Check sheet for the modelled part. Datum: model origin and axes. Units: mm. Face numbers are marked on the shaded views. A direction names the side the tool comes from. Round coordinates to 2 decimals unless told otherwise and drop trailing zeros. Write each loop counter-clockwise with the first axis right and the second up, starting at its lowest first coordinate (ties: lowest second). Pieces come first, ordered by that corner, then holes. Notation, with made-up numbers: (11.5, 14.25) - (18.5, 14.25) arc R4 ccw to (18.5, 19.25) - close; hole circle Ø3 at (32, 76). An arc over 180 degrees is marked (long way). Answer as a JSON object with one key per item and string values. Group by question number.
Item 1: Sectioned sample at D-D on y = 7.25. Record the boundary of the cut face in (x, z), plus the area to 3 significant figures.
Item 2: Set-up check for the marked faces 1, 2 and 3: record each of +Z, -Z, +X, -X, +Y, -Y from which the full face is reachable in a straight line by a thin tool's end or side.
Item 3: Thickness scan on line 1 (X direction, y = 14, z = -38); line 2 (X direction, y = 11.5, z = -36); line 3 (Z direction, x = 34, y = 10.5). Record the ranges inside material, lowest first.
Item 4: Sectioned sample at A-A on y = 1. Record the boundary of the cut face in (x, z) (1 decimal), plus the area to 3 significant figures.
Item 5: Sectioned sample at B-B on z = -20. Record the boundary of the cut face in (x, y) (1 decimal), plus the area to 3 significant figures.
Item 6: Sectioned sample at C-C on x = 13.5. Record the boundary of the cut face in (y, z) (3 decimals), plus the area to 4 significant figures.
Item 7: Gauge pin test, flat ends, axial feed: P1, Ø5, axis at x = 51, y = 11, coming from the -Z side; P2, Ø6.5, axis at y = 7.5, z = -39, coming from the +X side; P3, Ø6.5, axis at x = 49.5, y = 11, coming from the +Z side. Record the tip position at first contact, or that the pin passes through.
```python
from build123d import *

# Parameters (mm, degrees)
SKETCH1_W               = 79.375
SKETCH1_H               = 79.375
BOSS_EXTRUDE1_DEPTH     = 4
SKETCH2_W               = 43.02
SKETCH2_H               = 43.02
SKETCH2_R               = 5.461
BOSS_EXTRUDE2_DEPTH     = 11
SKETCH3_R               = 5.461
CUT_EXTRUDE1_DEPTH      = 1
CUT_EXTRUDE1_DEPTH_BACK = 16
SKETCH4_W               = 38.805624494
SKETCH4_H               = 17.902161279
SKETCH4_W_2             = 9.122
SKETCH4_H_2             = 9.122
BOSS_EXTRUDE3_DEPTH     = 15


with BuildPart() as part:
    # Sketch1 → Boss-Extrude1 (new body)
    with BuildSketch(Plane(origin=(0, 0, 0), x_dir=(1, 0, 0), z_dir=(0, 1, 0))):
        with Locations((39.6875, 39.6875)):
            Rectangle(SKETCH1_W, SKETCH1_H)
    extrude(amount=BOSS_EXTRUDE1_DEPTH)

    # Sketch2 → Boss-Extrude2 (add)
    with BuildSketch(Plane(origin=(0, 4, 0), x_dir=(1, 0, 0), z_dir=(0, 1, 0))):
        with Locations((39.6875, 39.6875)):
            Rectangle(SKETCH2_W, SKETCH2_H)
        with Locations((28.6385, 39.6875)):
            Circle(SKETCH2_R, mode=Mode.SUBTRACT)
        with Locations((50.7365, 39.6875)):
            Circle(SKETCH2_R, mode=Mode.SUBTRACT)
    extrude(amount=BOSS_EXTRUDE2_DEPTH)

    # Sketch3 → Cut-Extrude1 (cut, two sides)
    with BuildSketch(Plane(origin=(0, 15, 0), x_dir=(1, 0, 0), z_dir=(0, 1, 0))) as cut_extrude1_sk:
        with Locations((28.6385, 39.6875)):
            Circle(SKETCH3_R)
        with Locations((50.7365, 39.6875)):
            Circle(SKETCH3_R)
    extrude(amount=CUT_EXTRUDE1_DEPTH, mode=Mode.SUBTRACT)
    extrude(cut_extrude1_sk.sketch, amount=-CUT_EXTRUDE1_DEPTH_BACK, mode=Mode.SUBTRACT)

    # Sketch4 → Boss-Extrude3 (add)
    with BuildSketch(Plane(origin=(0, 15, 0), x_dir=(1, 0, 0), z_dir=(0, 1, 0))):
        with Locations((39.727968959, 38.830978853)):
            Rectangle(SKETCH4_W, SKETCH4_H)
        with Locations((28.6385, 39.6875)):
            Rectangle(SKETCH4_W_2, SKETCH4_H_2, mode=Mode.SUBTRACT)
        with Locations((50.7365, 39.6875)):
            Rectangle(SKETCH4_W_2, SKETCH4_H_2, mode=Mode.SUBTRACT)
    extrude(amount=-BOSS_EXTRUDE3_DEPTH)


solid = part.part
```
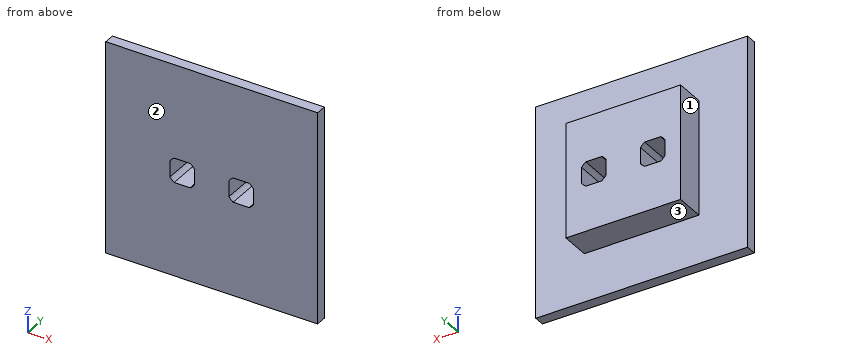
Completed:
{
 "1": {"outline": "(18.18, -61.2) - (61.2, -61.2) - (61.2, -18.18) - (18.18, -18.18) - close; hole (24.08, -42.69) arc R5.46 ccw to (25.64, -44.25) - (31.64, -44.25) arc R5.46 ccw to (33.2, -42.69) - (33.2, -36.68) arc R5.46 ccw to (31.64, -35.13) - (25.64, -35.13) arc R5.46 ccw to (24.08, -36.68) - close; hole (46.18, -42.69) arc R5.46 ccw to (47.73, -44.25) - (53.74, -44.25) arc R5.46 ccw to (55.3, -42.69) - (55.3, -36.68) arc R5.46 ccw to (53.74, -35.13) - (47.73, -35.13) arc R5.46 ccw to (46.18, -36.68) - close", "area": "1,690 mm²"},
 "2": {"face 1": "+Z, -Z, -X, +Y", "face 2": "+Z, -Z, +X, -X, -Y", "face 3": "-Z, +X, -X, +Y"},
 "3": {"line 1": "18.18 to 24.08, 33.2 to 46.18, 55.3 to 61.2", "line 2": "18.18 to 24.61, 32.67 to 46.71, 54.76 to 61.2", "line 3": "-61.2 to -18.18"},
 "4": {"outline": "(0, -79.4) - (79.4, -79.4) - (79.4, 0) - (0, 0) - close; hole (24.1, -42.7) arc R5.5 ccw to (25.6, -44.2) - (31.6, -44.2) arc R5.5 ccw to (33.2, -42.7) - (33.2, -36.7) arc R5.5 ccw to (31.6, -35.1) - (25.6, -35.1) arc R5.5 ccw to (24.1, -36.7) - close; hole (46.2, -42.7) arc R5.5 ccw to (47.7, -44.2) - (53.7, -44.2) arc R5.5 ccw to (55.3, -42.7) - (55.3, -36.7) arc R5.5 ccw to (53.7, -35.1) - (47.7, -35.1) arc R5.5 ccw to (46.2, -36.7) - close", "area": "6,140 mm²"},
 "5": {"outline": "(0, 0) - (79.4, 0) - (79.4, 4) - (61.2, 4) - (61.2, 15) - (18.2, 15) - (18.2, 4) - (0, 4) - close", "area": "791 mm²"},
 "6": {"outline": "(0, -79.375) - (4, -79.375) - (4, 0) - (0, 0) - close", "area": "317.5 mm²"},
 "7": {"P1": "z = -61.2", "P2": "x = 61.2", "P3": "z = -18.18"}
}
